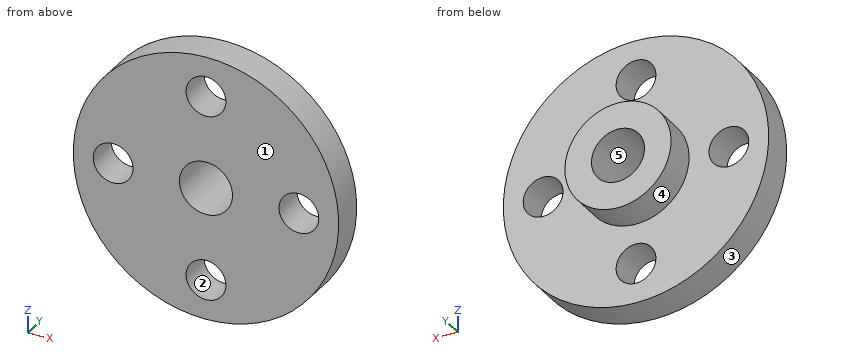
from build123d import *

# Parameters (mm, degrees)
SKETCH_1_R          = 10
SKETCH_1_R_2        = 2
EXTRUDE_1_DEPTH     = 2.5
SKETCH_2_R          = 4
SKETCH_2_R_2        = 2
EXTRUDE_2_DEPTH     = 2.5
SKETCH_3_R          = 1.5
CUT_EXTRUDE_1_DEPTH = 2.5


with BuildPart() as part:
    # 草图1 → 凸台-拉伸1 (new body)
    with BuildSketch(Plane(origin=(0, 0, 0), x_dir=(1, 0, 0), z_dir=(0, 1, 0))):
        with Locations(Location((0, 0, 0), (0, 0, 270))):
            Circle(SKETCH_1_R)
        with Locations(Location((0, 0, 0), (0, 0, 270))):
            Circle(SKETCH_1_R_2, mode=Mode.SUBTRACT)
    extrude(amount=EXTRUDE_1_DEPTH)

    # 草图2 → 凸台-拉伸2 (add)
    with BuildSketch(Plane(origin=(0, 2.5, 0), x_dir=(1, 0, 0), z_dir=(0, 1, 0))):
        with Locations(Location((0, 0, 0), (0, 0, 270))):
            Circle(SKETCH_2_R)
        with Locations(Location((0, 0, 0), (0, 0, 270))):
            Circle(SKETCH_2_R_2, mode=Mode.SUBTRACT)
    extrude(amount=EXTRUDE_2_DEPTH)

    # 草图3 → 切除-拉伸1 (cut)
    with BuildSketch(Plane(origin=(0, 2.5, 0), x_dir=(1, 0, 0), z_dir=(0, 1, 0))):
        with Locations(Location((0, 7, 0), (0, 0, 270))):
            Circle(SKETCH_3_R)
        with Locations(Location((7, 0, 0), (0, 0, 270))):
            Circle(SKETCH_3_R)
        with Locations(Location((0, -7, 0), (0, 0, 270))):
            Circle(SKETCH_3_R)
        with Locations(Location((-7, 0, 0), (0, 0, 270))):
            Circle(SKETCH_3_R)
    extrude(amount=-CUT_EXTRUDE_1_DEPTH, mode=Mode.SUBTRACT)


solid = part.part
Could you check a few things on this model? Use its own coordinates, in mm. Face numbers are marked on the shaded views. A direction names the side the tool comes from. Round coordinates to 2 decimals unless told otherwise and drop trailing zeros. Order: outer loops, then holes, each group sorted by start corner. A loop starts at its lowest first (then second) coordinate and runs counter-clockwise, first axis right, second up.
(1) Imagine slicing it at B-B (x = -1.75). Write out the boundary of the cut face in (y, z), plus the area to 3 significant figures.
Response values:
outline: (0, -9.85) - (2.5, -9.85) - (2.5, -3.6) - (5, -3.6) - (5, -0.97) - (0, -0.97) - close; (0, 0.97) - (5, 0.97) - (5, 3.6) - (2.5, 3.6) - (2.5, 9.85) - (0, 9.85) - close
area: 57.5 mm2
(2) Imagine slicing it at A-A (z = 0). Write out the boundary of the cut face in (x, y), plus the area to 3 significant figures.
Response values:
outline: (-10, 0) - (-8.5, 0) - (-8.5, 2.5) - (-10, 2.5) - close; (-5.5, 0) - (-2, 0) - (-2, 5) - (-4, 5) - (-4, 2.5) - (-5.5, 2.5) - close; (2, 0) - (5.5, 0) - (5.5, 2.5) - (4, 2.5) - (4, 5) - (2, 5) - close; (8.5, 0) - (10, 0) - (10, 2.5) - (8.5, 2.5) - close
area: 35.0 mm2
(3) Imagine slicing it at D-D (z = 7). Write out the boundary of the cut face in (x, y).
Response values:
outline: (-7.14, 0) - (-1.5, 0) - (-1.5, 2.5) - (-7.14, 2.5) - close; (1.5, 0) - (7.14, 0) - (7.14, 2.5) - (1.5, 2.5) - close
(4) Please list where these lines run through material, in increasing order: line 1 along X through (y, z) = (1.3, 0); line 2 along X through (y, z) = (2.9, 0); line 3 along Z through (x, y) = (-5.75, 0.35).
Response values:
line 1: x = -10 to -8.5, -5.5 to -2, 2 to 5.5, 8.5 to 10
line 2: x = -4 to -2, 2 to 4
line 3: z = -8.18 to -0.83, 0.83 to 8.18
(5) Imagine slicing it at C-C (y = 1.65). Write out the boundary of the cut face in (x, z), plus the area to 3 significant figures.
Response values:
outline: circle Ø20 at (0, 0); hole circle Ø3 at (-7, 0); hole circle Ø4 at (0, 0); hole circle Ø3 at (0, -7); hole circle Ø3 at (0, 7); hole circle Ø3 at (7, 0)
area: 273 mm2
(6) I'm going to push flat-ended pins straight in: pin 1 (4 mm diameter, centred on x = 0, z = 7, fed in from +Y); pin 2 (1.5 mm diameter, centred on x = 1, y = 1, fed in from +Z); pin 3 (1 mm diameter, centred on x = -4, y = 3.5, fed in from -Z). Where does each tip first touch, or does it pass through?
Response values:
pin 1: stops at y = 2.5
pin 2: stops at z = 10
pin 3: stops at z = -1.94
(7) If we mould it in two halves opening along Z, with no side actions, what happens to the marked faces 1, 2 and 3? For each: released by +Z, released by -Z, zero draft, split by the parting line, or undercut.
Response values:
face 1: zero draft
face 2: undercut
face 3: split by the parting line
(8) Which directions (+Z, -Z, +X, -X, +Y, -Y) give clear straight access to the entire face, cutting with the end or side of a thin tool? Please do the marked faces 4 and 5.
Response values:
face 4: +Y
face 5: +Y, -Y
